from build123d import *

# Parameters (mm, degrees)
SKETCH1_W           = 83.82
SKETCH1_H           = 7.62
BOSS_EXTRUDE1_DEPTH = 101.6
SKETCH1_3_W         = 36.399658141
SKETCH1_3_H         = 11.700173665
BOSS_EXTRUDE2_DEPTH = 7.62
SKETCH2_R           = 2.54
CUT_EXTRUDE1_DEPTH  = 112.58977198
SKETCH4_R           = 2.342393744
SKETCH4_R_2         = 1.801613949
SKETCH4_R_3         = 2.035024278
SKETCH4_R_4         = 2.216848317
CUT_EXTRUDE2_DEPTH  = 111.993574531


with BuildPart() as part:
    # Sketch1 → Boss-Extrude1 (new body)
    with BuildSketch(Plane(origin=(0, 0, 0), x_dir=(1, 0, 0), z_dir=(0, 1, 0))):
        Rectangle(SKETCH1_W, SKETCH1_H)
    extrude(amount=BOSS_EXTRUDE1_DEPTH)

    # Sketch1_3 → Boss-Extrude2 (add)
    with BuildSketch(Plane(origin=(0, 0, 0), x_dir=(1, 0, 0), z_dir=(0, 1, 0))):
        with Locations((-0.402628594, 9.660086833)):
            Rectangle(SKETCH1_3_W, SKETCH1_3_H)
    extrude(amount=BOSS_EXTRUDE2_DEPTH)

    # Sketch2 → Cut-Extrude1 (cut, through all)
    with BuildSketch(Plane.XY.offset(3.81)):
        with Locations((-23.8252, 59.901607654)):
            Circle(SKETCH2_R)
        with Locations((31.13358591, 88.819007782)):
            Circle(SKETCH2_R)
        with Locations((1.896113018, 39.534948803)):
            Circle(SKETCH2_R)
        with Locations((35.914623783, 12.5984)):
            Circle(SKETCH2_R)
        with Locations((35.914623783, 32.9184)):
            Circle(SKETCH2_R)
        Polygon((-41.91, 45.084065347), (-6.353580499, 101.6), (-41.91, 101.6), align=None)
        Polygon((-41.91, 38.321571432), (-11.466633524, 31.542928235), (-7.95768881, 0), (-41.91, 0), align=None)
    extrude(amount=-CUT_EXTRUDE1_DEPTH, mode=Mode.SUBTRACT)

    # Sketch4 → Cut-Extrude2 (cut, through all)
    with BuildSketch(Plane.XZ):
        with Locations(Location((4.32420412, -4.873516041, 0), (0, 0, 270))):
            Circle(SKETCH4_R)
        with Locations(Location((-1.801613949, -9.872883882, 0), (0, 0, 270))):
            Circle(SKETCH4_R_2)
        with Locations((-11.131176948, -7.373516021)):
            Circle(SKETCH4_R_3)
        with Locations((-14.801613949, -10.542756863)):
            Circle(SKETCH4_R_4)
    extrude(amount=-CUT_EXTRUDE2_DEPTH, mode=Mode.SUBTRACT)


solid = part.part
Here's how the part is built. I have some questions about the finished solid (model axes, mm). Round coordinates to 2 decimals unless told otherwise and drop trailing zeros. Loops run counter-clockwise (first coordinate to the right, second up) from the corner with the lowest first, then second, coordinate; pieces in that order, holes last. Notation, with made-up numbers: (63.25, 49.5) - (89.25, 49.5) arc R17 ccw to (89.25, 63.5) - close; hole circle Ø11 at (55.25, 81). An arc over 180 degrees is marked (long way). One line per question, with ' | ' between items. Start each with the question number.
Q1. I want a section at C-C (y = 56). Write out the boundary of the cut face in (x, z).
Q2. We'd pull the mould along X, two halves only. Please class faces 1 (the flat face through (17.797, 4, -10)), 2 (the flat face through (4, 7.62, -10)), 3 (the cylindrical face through (28.596, 88.931, 0.053)), 4 (the flat face through (-9.347, 12.487, -1.421)): +X half, -X half, draft (parallel to the pull), parting line (faces both ways), or undercut.
Q3. Please list where these lines run through material, in increasing order: line 1 (Y direction, x = -4, z = -7); line 2 (X direction, y = 10.5, z = -0.5); line 3 (Z direction, x = 15, y = 10). Write a range as [from, to].
Q4. I want a section at A-A (z = -9.25). Write out the boundary of the cut face in (x, y), then the cut area to 3 significant figures.
Q5. Will these pins go through, and if not, where does the flat tip stop? pin 1 (2 mm diameter, centred on x = 18.5, z = -11, fed in from -Y); pin 2 (8 mm diameter, centred on x = 19, y = 51, fed in from -Z); pin 3 (6 mm diameter, centred on x = -1.8, z = -9.87, fed in from +Y); pin 4 (8.5 mm diameter, centred on y = 4, z = -10, fed in from +X).
Q6. I want a section at B-B (x = 36). Write out the boundary of the cut face in (y, z).
Q7. I want a section at D-D (z = -0.75). Write out the boundary of the cut face in (x, y), then the cut area to 3 significant figures.
Response values:
1) outline: (-35.04, -3.81) - (2.24, -3.81) arc R2.34 cw to (6.41, -3.81) - (41.91, -3.81) - (41.91, 3.81) - (-35.04, 3.81) - close
2) face 1: +X half | face 2: draft | face 3: undercut | face 4: -X half
3) line 1: y = [0, 7.62] | line 2: x = [-9.13, 34.48], [37.35, 41.91] | line 3: z = [-3.81, 3.81]
4) outline: (-8.81, 7.62) - (-7.96, 0) - (-3.49, 0) - (-3.49, 7.62) - close; (-0.11, 0) - (17.8, 0) - (17.8, 7.62) - (-0.11, 7.62) - close | area: 174 mm²
5) pin 1: stops at y = 0 | pin 2: stops at z = -3.81 | pin 3: stops at y = 7.62 | pin 4: stops at x = 17.8
6) outline: (0, -3.81) - (10.06, -3.81) - (10.06, 3.81) - (0, 3.81) - close; (15.14, -3.81) - (30.38, -3.81) - (30.38, 3.81) - (15.14, 3.81) - close; (35.46, -3.81) - (101.6, -3.81) - (101.6, 3.81) - (35.46, 3.81) - close
7) outline: (-41.91, 38.32) - (-11.47, 31.54) - (-7.96, 0) - (41.91, 0) - (41.91, 101.6) - (-6.35, 101.6) - (-41.91, 45.08) - close; hole circle Ø5.08 at (-23.83, 59.9); hole circle Ø5.08 at (1.9, 39.53); hole circle Ø5.08 at (31.13, 88.82); hole circle Ø5.08 at (35.91, 12.6); hole circle Ø5.08 at (35.91, 32.92) | area: 6,290 mm²
